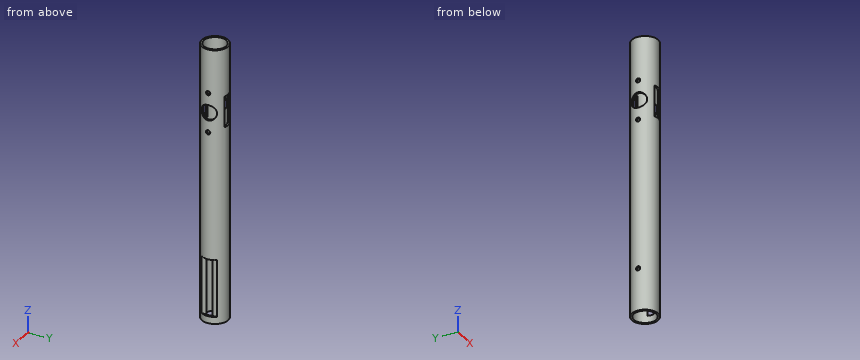
```python
from build123d import *

# Parameters (mm, degrees)
SKETCH1_R           = 9.36
SKETCH1_R_2         = 7.99
EXTRUDE1_DEPTH      = 195
SKETCH2_R           = 1.5
SKETCH2_R_2         = 5.5
EXTRUDE2_DEPTH      = 10.36
EXTRUDE2_DEPTH_BACK = 10.36
SKETCH3_W           = 6.35
SKETCH3_H           = 40.5
SKETCH3_W_2         = 7
SKETCH3_H_2         = 22
EXTRUDE3_DEPTH      = 25
EXTRUDE3_DEPTH_BACK = 25


with BuildPart() as part:
    # Sketch1 → Extrude1 (new body)
    with BuildSketch(Plane.XY):
        Circle(SKETCH1_R)
        Circle(SKETCH1_R_2, mode=Mode.SUBTRACT)
    extrude(amount=EXTRUDE1_DEPTH)

    # Sketch2 → Extrude2 (cut, two sides)
    with BuildSketch(Plane(origin=(0, 0, 0), x_dir=(0, 0, -1), z_dir=(1, 0, 0))) as extrude2_sk:
        with Locations((-30, 0)):
            Circle(SKETCH2_R)
        with Locations((-150, 0)):
            Circle(SKETCH2_R_2)
        with Locations((-136.0625, 0)):
            Circle(SKETCH2_R)
        with Locations((-163.9375, 0)):
            Circle(SKETCH2_R)
    extrude(amount=EXTRUDE2_DEPTH, mode=Mode.SUBTRACT)
    extrude(extrude2_sk.sketch, amount=-EXTRUDE2_DEPTH_BACK, mode=Mode.SUBTRACT)

    # Sketch3 → Extrude3 (cut, two sides)
    with BuildSketch(Plane(origin=(0, 0, 0), x_dir=(1, 0, 0), z_dir=(0, 1, 0))) as extrude3_sk:
        with Locations((10.875, -25.25)):
            Rectangle(SKETCH3_W, SKETCH3_H)
        with Locations((0, -150)):
            Rectangle(SKETCH3_W_2, SKETCH3_H_2)
    extrude(amount=EXTRUDE3_DEPTH, mode=Mode.SUBTRACT)
    extrude(extrude3_sk.sketch, amount=-EXTRUDE3_DEPTH_BACK, mode=Mode.SUBTRACT)


solid = part.part
```
For this review, take the finished solid that the model builds, in its own axes (mm). Round coordinates to 2 decimals unless told otherwise and drop trailing zeros. Write each loop counter-clockwise with the first axis right and the second up, starting at its lowest first coordinate (ties: lowest second). Pieces come first, ordered by that corner, then holes. Notation, with made-up numbers: (-6, 18) - (52, 18) arc R22 cw to (52, 31) - close; hole circle Ø11 at (38.25, -10.75). An arc over 180 degrees is marked (long way). Put each result on its own line as item: value.
Q1. We need section D-D (z = 52.5). Give the boundary of the cut face in (x, y).
Solved:
outline: circle Ø18.72 at (0, 0); hole circle Ø15.98 at (0, 0)
Q2. Insertion check: pin 1 Ø6 at (x, z) = (-3, 151.5) entering from +Y; pin 2 Ø2.5 at (y, z) = (4, 20) entering from +X; pin 3 Ø0.7 at (y, z) = (8.5, 150.5) entering from +X; pin 4 Ø10 at (y, z) = (0, 150) entering from -X. Each pin has a flat end and moves straight along its axis. Give the tip position at first contact, or say it passes through.
Solved:
pin 1: stops at y = 8.68
pin 2: stops at x = 7.7
pin 3: stops at x = 4.6
pin 4: passes through
Q3. We need section C-C (z = 22). Give the boundary of the cut face in (x, y).
Solved:
outline: (7.7, -5.32) - (7.7, -2.13) arc R7.99 cw (long way) to (7.7, 2.13) - (7.7, 5.32) arc R9.36 ccw (long way) to start
Q4. We need section B-B (z = 150). Give the boundary of the cut face in (x, y).
Solved:
outline: (-7.57, -5.5) arc R9.36 ccw to (-3.5, -8.68) - (-3.5, -7.18) arc R7.99 cw to (-5.8, -5.5) - close; (-7.57, 5.5) - (-5.8, 5.5) arc R7.99 cw to (-3.5, 7.18) - (-3.5, 8.68) arc R9.36 ccw to start; (3.5, -8.68) arc R9.36 ccw to (7.57, -5.5) - (5.8, -5.5) arc R7.99 cw to (3.5, -7.18) - close; (3.5, 7.18) arc R7.99 cw to (5.8, 5.5) - (7.57, 5.5) arc R9.36 ccw to (3.5, 8.68) - close
Q5. We need section A-A (x = 0). Give the boundary of the cut face in (y, z), and give its area (3 significant figures).
Solved:
outline: (-9.36, 0) - (-7.99, 0) - (-7.99, 139) - (-9.36, 139) - close; (-9.36, 161) - (-7.99, 161) - (-7.99, 195) - (-9.36, 195) - close; (7.99, 0) - (9.36, 0) - (9.36, 139) - (7.99, 139) - close; (7.99, 161) - (9.36, 161) - (9.36, 195) - (7.99, 195) - close
area: 474 mm2
Q6. Wall thickness on probe 1 along Y at (x, z) = (0, 78); probe 2 along Y at (x, z) = (2, 40): over which ranges is each line inside the solid? List them lowest first.
Solved:
probe 1: y = -9.36 to -7.99, 7.99 to 9.36
probe 2: y = -9.14 to -7.74, 7.74 to 9.14
